from build123d import *

# Parameters (mm, degrees)
SKETCH1_W                      = 5
SKETCH1_H                      = 25
BOSS_EXTRUDE1_DEPTH            = 10
BOSS_EXTRUDE2_DEPTH            = 2.5
BOSS_EXTRUDE3_START            = 2.5
BOSS_EXTRUDE3_DEPTH            = 2.5
SKETCH5_W                      = 50
SKETCH5_H                      = 44
SKETCH5_R                      = 1.65
BOSS_EXTRUDE4_DEPTH            = 5
DRAFT1_ANGLE                   = 60
DRAFT2_ANGLE                   = -10
SKETCH6_W                      = 5
SKETCH6_H                      = 15
SKETCH7_W                      = 5
SKETCH7_H                      = 15
SKETCH8_W                      = 5
SKETCH8_H                      = 25
F_10_0_10_DIAMETER_HOLE1_D     = 10
F_10_0_10_DIAMETER_HOLE1_DEPTH = 29.5
FILLET1_R                      = 5
FILLET2_R                      = 20
FILLET3_R                      = 15


with BuildPart() as part:
    # Sketch1 → Revolve1 (revolve)
    with BuildSketch(Plane(origin=(0, -7.5, 0), x_dir=(1, 0, 0), z_dir=(0, 1, 0))):
        with Locations((-5.811233855, 90.876419512)):
            Rectangle(SKETCH1_W, SKETCH1_H)
    revolve(axis=Axis((-8.311233855, -7.5, -103.376419512), (0, 0, 1)))

    # Sketch2 → Boss-Extrude1 (add)
    with BuildSketch(Plane(origin=(0, -2.5, 0), x_dir=(1, 0, 0), z_dir=(0, 1, 0))):
        with BuildLine():
            Line((-20.904218066, -4.060593221), (-17.745761276, -10))
            ThreePointArc((-17.745761276, -10), (-16.42436709, -8.86625844), (-15.571850751, -7.348145002))
            Line((-15.571850751, -7.348145002), (-13.235172111, -0.671920317))
            ThreePointArc((-13.235172111, -0.671920317), (-13.124251068, -0.312083076), (-13.040724348, 0.055081199))
            ThreePointArc((-13.040724348, 0.055081199), (-9.034250588, -1.999882688), (-5, 0))
            ThreePointArc((-5, 0), (-1.464466094, 1.464466094), (0, 5))
            Line((0, 5), (0, 35))
            ThreePointArc((0, 35), (-10.533604853, 36.723434751), (-20.057952451, 41.541511272))
            Line((-20.057952451, 41.541511272), (5.197843412, 71.090018979))
            Line((5.197843412, 71.090018979), (8.982632418, 71.090018979))
            Line((8.982632418, 71.090018979), (8.982632418, 78.376419512))
            Line((8.982632418, 78.376419512), (-8.311233855, 78.376419512))
            Line((-8.311233855, 78.376419512), (-41.017367582, 78.376419512))
            Line((-41.017367582, 78.376419512), (-54.819345863, 40.83303933))
            Line((-54.819345863, 40.83303933), (-54.896976862, 16.766177236))
            ThreePointArc((-54.896976862, 16.766177236), (-54.712461515, 16.524099343), (-54.430876141, 16.639673113))
            Line((-54.430876141, 16.639673113), (-49.872077715, 24.477250263))
            Line((-49.872077715, 24.477250263), (-8.967847829, 0.684930874))
            Line((-8.967847829, 0.684930874), (-28.967743782, 0.74944331))
            Line((-28.967743782, 0.74944331), (-28.987601327, -5.406715976))
            ThreePointArc((-28.987601327, -5.406715976), (-28.311946244, -7.932877153), (-26.453503439, -9.772494077))
            Line((-26.453503439, -9.772494077), (-20.904218066, -4.060593221))
        make_face()
    extrude(amount=-BOSS_EXTRUDE1_DEPTH)

    # Sketch3 → Boss-Extrude2 (add)
    with BuildSketch(Plane.XZ.offset(12.5)):
        with BuildLine():
            Line((-20.904218066, 4.060593221), (-17.745761276, 10))
            ThreePointArc((-17.745761276, 10), (-16.42436709, 8.86625844), (-15.571850751, 7.348145002))
            Line((-15.571850751, 7.348145002), (-13.235172111, 0.671920317))
            ThreePointArc((-13.235172111, 0.671920317), (-13.124251068, 0.312083076), (-13.040724348, -0.055081199))
            ThreePointArc((-13.040724348, -0.055081199), (-9.034250588, 1.999882688), (-5, 0))
            ThreePointArc((-5, 0), (-1.464466094, -1.464466094), (0, -5))
            Line((0, -5), (0, -35))
            ThreePointArc((0, -35), (-10.533604853, -36.723434751), (-20.057952451, -41.541511272))
            Line((-20.057952451, -41.541511272), (5.197843412, -71.090018979))
            Line((5.197843412, -71.090018979), (8.982632418, -71.090018979))
            Line((8.982632418, -71.090018979), (8.982632418, -78.376419512))
            Line((8.982632418, -78.376419512), (-41.017367582, -78.376419512))
            Line((-41.017367582, -78.376419512), (-54.819345863, -40.83303933))
            Line((-54.819345863, -40.83303933), (-54.896976862, -16.766177236))
            ThreePointArc((-54.896976862, -16.766177236), (-54.712461515, -16.524099343), (-54.430876141, -16.639673113))
            Line((-54.430876141, -16.639673113), (-49.872077715, -24.477250263))
            Line((-49.872077715, -24.477250263), (-8.967847829, -0.684930874))
            Line((-8.967847829, -0.684930874), (-28.967743782, -0.74944331))
            Line((-28.967743782, -0.74944331), (-28.987601327, 5.406715976))
            ThreePointArc((-28.987601327, 5.406715976), (-28.311946244, 7.932877153), (-26.453503439, 9.772494077))
            Line((-26.453503439, 9.772494077), (-20.904218066, 4.060593221))
        make_face()
    extrude(amount=BOSS_EXTRUDE2_DEPTH)

    # Sketch4 → Boss-Extrude3 (add)
    with BuildSketch(Plane(origin=(0, -2.5, 0), x_dir=(-1, 0, 0), z_dir=(0, 1, 0)).offset(BOSS_EXTRUDE3_START)):
        with BuildLine():
            Line((20.904218066, 4.060593221), (26.453503439, 9.772494077))
            ThreePointArc((26.453503439, 9.772494077), (28.311946244, 7.932877153), (28.987601327, 5.406715976))
            Line((28.987601327, 5.406715976), (28.967743782, -0.74944331))
            Line((28.967743782, -0.74944331), (8.967847829, -0.684930874))
            Line((8.967847829, -0.684930874), (49.872077715, -24.477250263))
            Line((49.872077715, -24.477250263), (54.430876141, -16.639673113))
            ThreePointArc((54.430876141, -16.639673113), (54.712461515, -16.524099343), (54.896976862, -16.766177236))
            Line((54.896976862, -16.766177236), (54.819345863, -40.83303933))
            Line((54.819345863, -40.83303933), (41.017367582, -78.376419512))
            Line((41.017367582, -78.376419512), (-8.982632418, -78.376419512))
            Line((-8.982632418, -78.376419512), (-8.982632418, -71.090018979))
            Line((-8.982632418, -71.090018979), (-5.197843412, -71.090018979))
            Line((-5.197843412, -71.090018979), (20.057952451, -41.541511272))
            ThreePointArc((20.057952451, -41.541511272), (10.533604853, -36.723434751), (0, -35))
            Line((0, -35), (0, -5))
            ThreePointArc((0, -5), (1.464466094, -1.464466094), (5, 0))
            ThreePointArc((5, 0), (9.034250588, 1.999882688), (13.040724348, -0.055081199))
            ThreePointArc((13.040724348, -0.055081199), (13.124251068, 0.312083076), (13.235172111, 0.671920317))
            Line((13.235172111, 0.671920317), (15.571850751, 7.348145002))
            ThreePointArc((15.571850751, 7.348145002), (16.42436709, 8.86625844), (17.745761276, 10))
            Line((17.745761276, 10), (20.904218066, 4.060593221))
        make_face()
    extrude(amount=-BOSS_EXTRUDE3_DEPTH)

    # Sketch5 → Boss-Extrude4 (add)
    with BuildSketch(Plane.XY.offset(-103.376419512)):
        with Locations((-14.91763051, -7.5)):
            Rectangle(SKETCH5_W, SKETCH5_H)
        with Locations((-29.91763051, -19.5)):
            Circle(SKETCH5_R, mode=Mode.SUBTRACT)
        with Locations((0.08236949, -19.5)):
            Circle(SKETCH5_R, mode=Mode.SUBTRACT)
        with Locations((0.08236949, 4.5)):
            Circle(SKETCH5_R, mode=Mode.SUBTRACT)
        with Locations((-29.91763051, 4.5)):
            Circle(SKETCH5_R, mode=Mode.SUBTRACT)
    extrude(amount=-BOSS_EXTRUDE4_DEPTH)

    # Draft1
    draft1_faces = [part.faces().sort_by_distance(p)[0] for p in [
        (-18.967795805, -7.5, -0.717187092),
    ]]
    draft(draft1_faces, Plane(origin=(-28.967743782, -12.5, -0.74944331), x_dir=(0.0032256218002524395, 0, -0.9999947976684688), z_dir=(-0.9999947976684688, 0, -0.0032256218002524395)), DRAFT1_ANGLE)

    # Draft2
    draft2_faces = [part.faces().sort_by_distance(p)[0] for p in [
        (8.982632418, -7.5, -74.733219246),
    ]]
    draft(draft2_faces, Plane(origin=(-8.311233855, -12.5, -78.376419512), x_dir=(-1, 0, 0), z_dir=(0, 0, -1)), DRAFT2_ANGLE)

    # Sketch6 → Cut-Revolve1 (revolve, cut)
    with BuildSketch(Plane.XY.offset(7)):
        with Locations((-19.5, -7.5)):
            Rectangle(SKETCH6_W, SKETCH6_H)
    revolve(axis=Axis((-22, 0, 7), (0, -1, 0)), mode=Mode.SUBTRACT)

    # Sketch7 → Cut-Revolve2 (revolve, cut)
    with BuildSketch(Plane(origin=(0, 0, -3), x_dir=(-1, 0, 0), z_dir=(0, 0, -1))):
        with Locations((6.5, -7.5)):
            Rectangle(SKETCH7_W, SKETCH7_H)
    revolve(axis=Axis((-9, -15, -3), (0, 1, 0)), mode=Mode.SUBTRACT)

    # Sketch8 → Revolve2 (revolve)
    with BuildSketch(Plane(origin=(0, -7.5, 0), x_dir=(1, 0, 0), z_dir=(0, 1, 0))):
        with Locations((-18.311233855, 90.876419512)):
            Rectangle(SKETCH8_W, SKETCH8_H)
    revolve(axis=Axis((-20.811233855, -7.5, -103.376419512), (0, 0, 1)))

    # Sketch9 → Revolve3 (revolve)
    with BuildSketch(Plane(origin=(0, -7.5, 0), x_dir=(1, 0, 0), z_dir=(0, 1, 0))):
        Polygon((-51.129054889, 22.316230044), (-52.386032062, 20.155209826), (-26.453789436, 5.071483748), (-25.196812263, 7.232503967), align=None)
    revolve(axis=Axis((-53.325247092, -7.5, -20.701512837), (0.8644080875330462, 0, 0.502790869256256)))

    # Ø10.0 (10) Diameter Hole1
    with Locations(Plane(origin=(0, -15, 0), x_dir=(-1, 0, 0), z_dir=(0, -1, 0))):
        with Locations((-0.318427602, 69.998551454)):
            Hole(F_10_0_10_DIAMETER_HOLE1_D / 2, depth=F_10_0_10_DIAMETER_HOLE1_DEPTH)

    # Chamfer1
    # the kernel refuses this chamfer: 0.262951912, 0.262770817 mm, written as the material it takes off along each edge
    with BuildSketch(Plane(origin=(-5, -15.679311202, 0), x_dir=(0.9996632496701223, 4.862291359988254e-15, -0.02594970633688609), z_dir=(0, 1, 0))) as chamfer1_piece_1:
        with BuildLine():
            Line((0.259497063, 0), (0.159812325, 0.213399124))
            ThreePointArc((0.159812325, 0.213399124), (0.082816569, 0.107621918), (0, 0))
            ThreePointArc((0, 0), (0.131972937, -0.001683257), (0.259497063, 0))
        make_face()
    extrude(amount=16.358622404, mode=Mode.SUBTRACT)

    # Fillet1
    fillet1_edges = [part.edges().sort_by_distance(p)[0] for p in [
        (-28.967743782, -7.5, -0.74944331),
        (8.982632418, -7.5, -78.376419512),
    ]]
    fillet(fillet1_edges, radius=FILLET1_R)

    # Fillet2
    fillet2_edges = [part.edges().sort_by_distance(p)[0] for p in [
        (-41.017367582, -7.5, -78.376419512),
        (-54.819345863, -7.5, -40.83303933),
    ]]
    fillet(fillet2_edges, radius=FILLET2_R)

    # Fillet3
    fillet3_edges = [part.edges().sort_by_distance(p)[0] for p in [
        (-39.91763051, -29.5, -105.876419512),
        (-39.91763051, 14.5, -105.876419512),
        (10.08236949, 14.5, -105.876419512),
        (10.08236949, -29.5, -105.876419512),
    ]]
    fillet(fillet3_edges, radius=FILLET3_R)


solid = part.part
Could you check a few things on this model? Use its own coordinates, in mm. A direction names the side the tool comes from. Coordinates: 2 decimals unless noted, no trailing zeros. Write each loop counter-clockwise with the first axis right and the second up, starting at its lowest first coordinate (ties: lowest second). Pieces come first, ordered by that corner, then holes. Notation, with made-up numbers: (35.25, 25) - (65.25, 25) arc R16 ccw to (65.25, 39) - close; hole circle Ø8 at (50.25, 48). An arc over 180 degrees is marked (long way). Put each result on its own line as item: value. Start each with the question number.
Q1. I want a section at B-B on z = -98. Write out the boundary of the cut face in (x, y), plus the area to 3 significant figures.
Q2. I want a section at C-C on y = -19.5. Write out the boundary of the cut face in (x, z).
Q3. Which directions (+Z, -Z, +X, -X, +Y, -Y) give clear straight access to the entire face, cutting with the end or side of a thin tool? Please do faces 5 (the flat face through (-15, -7, -108.376)), 6 (the flat face through (-36.724, -7.395, -16.83)), 7 (the flat face through (-39.918, -8, -106)), 8 (the flat face through (6, -7, -71.09)), 9 (the cylindrical face through (-24.496, -4.121, -91.051)).
Q4. I want a section at D-D on x = -6.5. Write out the boundary of the cut face in (y, z).
Q5. Thinking about a two-plate mould opening in Z: for faces 1 (the cylindrical face through (-0.28, 2.89, -105.84)), 2 (the flat face through (-14.4, -7.4, 4)), 3 (the flat face through (-49.772, -7.395, -54.562)), 4 (the cylindrical face through (-10.68, -7.4, -36.77)), which applies, pulls with the +Z half, pulls with the -Z half, needs draft (parallel to the pull), parting line crosses it, or undercut?
Q6. Please list where these lines run through material, in increasing order: L1, parallel to Z at x = -16, y = -5.5; L2, parallel to Y at x = -51.5, z = -48.5; L3, parallel to X at y = 4, z = -106.
Q7. I'm going to push flat-ended pins straight in: P1, Ø1.2, axis at x = 7, y = -4.5, coming from the +Z side; P2, Ø7.5, axis at y = -7, z = -24, coming from the +X side; P3, Ø6, axis at x = -22, z = 7, coming from the +Y side; P4, Ø12, axis at x = -11, z = -19, coming from the -Y side. Where does each tip first touch, or does it pass through?
Q8. I want a section at A-A on x = 6.5. Write out the boundary of the cut face in (y, z), plus the area to 3 significant figures.
Checks:
1. outline: circle Ø10 at (-20.81, -7.5); circle Ø10 at (-8.31, -7.5)
1. area: 157 mm²
2. outline: (-39.06, -108.38) - (-31.57, -108.38) - (-31.57, -103.38) - (-39.06, -103.38) - close; (-28.27, -108.38) - (-1.57, -108.38) - (-1.57, -103.38) - (-28.27, -103.38) - close; (1.73, -108.38) - (9.22, -108.38) - (9.22, -103.38) - (1.73, -103.38) - close
3. face 5: -Z, +X, -X, +Y, -Y
3. face 6: +Y, -Y
3. face 7: -Z, -X, +Y, -Y
3. face 8: +Z, +X, +Y, -Y
3. face 9: none
4. outline: (-29.5, -108.38) - (14.5, -108.38) - (14.5, -103.38) - (-2.84, -103.38) - (-2.84, -78.38) - (0, -78.38) - (0, -57.4) - (-15, -57.4) - (-15, -78.38) - (-12.16, -78.38) - (-12.16, -103.38) - (-29.5, -103.38) - close; (-15, -35.67) - (0, -35.67) - (0, -7.33) - (-15, -7.33) - close
5. face 1: needs draft
5. face 2: pulls with the +Z half
5. face 3: pulls with the -Z half
5. face 4: undercut
6. L1: -108.38 to -103.38, -78.38 to -46.29, -39.04 to 8.26
6. L2: -15 to 0
6. L3: -39.23 to -31.49, -28.35 to -1.49, 1.65 to 9.39
7. P1: z = -71.09
7. P2: x = 0
7. P3: through
7. P4: y = -15
8. outline: (-24.23, -108.38) - (9.23, -108.38) - (9.23, -103.38) - (-24.23, -103.38) - close; (-15, -76.97) - (0, -76.97) - (0, -71.09) - (-15, -71.09) - close
8. area: 255 mm²
